CAD build for the part. Positions are in the model's coordinates, mm. A direction names the side the tool comes from. Give positions to 0.01 mm unless a question says otherwise; leave off trailing zeros. Loops run counter-clockwise (first coordinate to the right, second up) from the corner with the lowest first, then second, coordinate; pieces in that order, holes last. Notation, with made-up numbers: (0, 59.5) -> (41, 59.5) arc R22 cw to (41, 73.5) -> close; hole circle Ø3 at (-10.75, 48.25). An arc over 180 degrees is marked (long way). Use one line per item in the form item = value.
```python
from build123d import *

# Parameters (mm, degrees)
ENL_V_START             = 0.5
ENL_V_MAT_EXTRU_1_DEPTH = 3
CHANFREIN1_SIZE         = 1


with BuildPart() as part:
    # Esquisse1 → Révolution1 (revolve)
    with BuildSketch(Plane.XY, mode=Mode.PRIVATE) as r_volution1_sk:
        with BuildLine():
            Line((0, -15), (0, 2.5))
            ThreePointArc((0, 2.5), (-2.371708245, 2.115124735), (-4.5, 1))
            Line((-4.5, 1), (-4.5, 0))
            Line((-4.5, 0), (-2.5, 0))
            Line((-2.5, 0), (-2.5, -15))
            Line((-2.5, -15), (0, -15))
        make_face()
    revolve(r_volution1_sk.sketch.rotate(Axis((0, 16.1829806, 0), (0, -1, 0)), 270), axis=Axis((0, 16.1829806, 0), (0, -1, 0)))  # turned: the seam where the file's is

    # Esquisse2 → Enlèv. mat.-Extru.1 (cut, through all)
    with BuildSketch(Plane(origin=(0, 0, 0), x_dir=(1, 0, 0), z_dir=(0, 1, 0)).offset(ENL_V_START)):
        Polygon((0, 1.732050808), (-1.5, 0.866025404), (-1.5, -0.866025404), (0, -1.732050808), (1.5, -0.866025404), (1.5, 0.866025404), align=None)
    extrude(amount=ENL_V_MAT_EXTRU_1_DEPTH, mode=Mode.SUBTRACT)

    # Chanfrein1
    chanfrein1_edges = [part.edges().sort_by_distance(p)[0] for p in [
        (0, -15, -2.5),
    ]]
    chamfer(chanfrein1_edges, length=CHANFREIN1_SIZE)


solid = part.part
```
1. Cut at A-A, the plane y = 0.75. Write the cut outline in (x, z), then the cut area to 3 significant figures.
Result sheet:
outline = circle Ø9 at (0, 0); hole (-1.5, -0.87) -> (0, -1.73) -> (1.5, -0.87) -> (1.5, 0.87) -> (0, 1.73) -> (-1.5, 0.87) -> close
area = 55.8 mm^2
2. Tool access for faces 4 (the flat face through (-0.76, 1.411, 1.293)), 5 (the cylindrical face through (2.44, -7.1, -0.54)), 6 (the flat face through (0, -15, 0)): list every direction of +Z, -Z, +X, -X, +Y, -Y with a clear straight run to the whole face (end or side of a thin tool).
Result sheet:
face_4 = +Y
face_5 = -Y
face_6 = +Z, -Z, +X, -X, -Y
3. Cut at C-C, the plane y = -10. Write the cut outline in (x, z).
Result sheet:
outline = circle Ø5 at (0, 0)
4. Drop flat-ended pins along their axis: P1, Ø0.9, axis at y = 1.5, z = 0, coming from the -X side; P2, Ø1.5, axis at y = -1.5, z = 0, coming from the +X side; P3, Ø2, axis at x = -3, y = -4.5, coming from the +Z side. Give the stop position or say it passes through.
Result sheet:
P1 = -4.43
P2 = 2.5
P3 = 1.5
5. Mould opens along X. For faces 1 (the cylindrical face through (-1.352, 0.493, 4.292)), 2 (the flat face through (0.74, 1.411, 1.305)), 3 (the flat face through (2, 0, 2)) say: pulls with the +X half, pulls with the -X half, needs draft (parallel to the pull), parting line crosses it, or undercut.
Result sheet:
face_1 = parting line crosses it
face_2 = undercut
face_3 = needs draft
6. Cut at B-B, the plane z = 0. Write the cut outline in (x, y), then the cut area to 3 significant figures.
Result sheet:
outline = (-4.5, 0) -> (-2.5, 0) -> (-2.5, -14) -> (-1.5, -15) -> (1.5, -15) -> (2.5, -14) -> (2.5, 0) -> (4.5, 0) -> (4.5, 1) arc R7.5 ccw to (1.5, 2.35) -> (1.5, 0.5) -> (-1.5, 0.5) -> (-1.5, 2.35) arc R7.5 ccw to (-4.5, 1) -> close
area = 86.3 mm^2
7. Cut at D-D, the plane x = -3.5. Write the cut outline in (y, z), then the cut area to 3 significant figures.
Result sheet:
outline = (0, -2.83) -> (1, -2.83) arc R6.63 ccw to (1, 2.83) -> (0, 2.83) -> close
area = 8.07 mm^2
8. Drill centre lines: line 1 (X direction, y = -10.5, z = -2); line 2 (Z direction, x = -0.5, y = 1.5); line 3 (Z direction, x = 1.75, y = -3.75). Where is each one in solid material? Low to high.
Result sheet:
line_1 = -1.5 to 1.5
line_2 = -3.71 to -1.44, 1.44 to 3.71
line_3 = -1.79 to 1.79
